from build123d import *

# Parameters (mm, degrees)
SKETCH1_R           = 6.25
SKETCH1_R_2         = 4
BOSS_EXTRUDE1_DEPTH = 15
BOSS_EXTRUDE2_START = 15
SKETCH1_3_R         = 4
BOSS_EXTRUDE2_DEPTH = 30
SKETCH2_R           = 2
CUT_EXTRUDE1_DEPTH  = 12


with BuildPart() as part:
    # Sketch1 → Boss-Extrude1 (new body)
    # profile 1 of 2: a face of its own
    with BuildSketch(Plane.XY):
        Circle(SKETCH1_R)
        Circle(SKETCH1_R_2, mode=Mode.SUBTRACT)
    # profile 2 of 2: a face of its own
    with BuildSketch(Plane.XY):
        Circle(SKETCH1_R_2)
    extrude(amount=BOSS_EXTRUDE1_DEPTH)

    # Sketch1<3> → Boss-Extrude2 (add)
    with BuildSketch(Plane.XY.offset(BOSS_EXTRUDE2_START)):
        Circle(SKETCH1_3_R)
    extrude(amount=BOSS_EXTRUDE2_DEPTH)

    # Sketch2 → Cut-Extrude1 (cut)
    with BuildSketch(Plane(origin=(0, 0, 0), x_dir=(-1, 0, 0), z_dir=(0, 0, -1))):
        Circle(SKETCH2_R)
    extrude(amount=-CUT_EXTRUDE1_DEPTH, mode=Mode.SUBTRACT)


solid = part.part
Part model, mm, in its own coordinate system. A direction names the side the tool comes from. Coordinates: 2 decimals unless noted, no trailing zeros. Loops run counter-clockwise (first coordinate to the right, second up) from the corner with the lowest first, then second, coordinate; pieces in that order, holes last. Notation, with made-up numbers: M 11.25,5 L 67.25,5 A21 ccw 67.25,23 Z; hole C 37,68.25 d3. An arc over 180 degrees is marked long. Use a Markdown table: item, result. Add a question column.
Q1. Cut at C-C (z = 9.5). Write the cut outline in (x, y), and give its area (3 significant figures).
Q2. Probe L1, parallel to Y at x = 0, z = 6.25; L2, parallel to Z at x = -4.25, y = 3.5; L3, parallel to Z at x = 0.75, y = -1.75. List the from-to ranges inside material, lowest first.
Q3. Which spindle directions (+Z, -Z, +X, -X, +Y, -Y) get a long thin tool onto all of the face, cutting with end or side? Do faces 1 (the flat face through (1.3, -4.1, 15)), 2 (the cylindrical face through (0, -2, 6)), 3 (the flat face through (0, -3, 0)). Say none if no direction does.
Q4. Cut at D-D (z = 35.5). Write the cut outline in (x, y), and give its area (3 significant figures).
Q5. Mould opens along X. For faces 4 (the flat face through (0, 0, 12)), 5 (the cylindrical face through (-0.867, -3.905, 29.79)), 6 (the flat face through (0, 0, 45)) say: +X half, -X half, draft (parallel to the pull), parting line (faces both ways), or undercut.
Q6. Cut at A-A (x = 0). Write the cut outline in (y, z), and give its area (4 significant figures).
Q7. Pin check, flat tips, straight feed: P1, Ø3, axis at x = -3, z = 24.5, coming from the -Y side; P2, Ø2, axis at y = -4.5, z = 16.5, coming from the +X side; P3, Ø4, axis at y = 0, z = 35.5, coming from the +X side. Stop position of each tip, or through.
Worked out:
| question | item | result |
|---|---|---|
| 1 | outline | C 0,0 d12.5; hole C 0,0 d4 |
| 1 | area | 110 mm2 |
| 2 | L1 | y = -6.25 to -2, 2 to 6.25 |
| 2 | L2 | z = 0 to 15 |
| 2 | L3 | z = 12 to 45 |
| 3 | face 1 | +Z |
| 3 | face 2 | -Z |
| 3 | face 3 | -Z, +X, -X, +Y, -Y |
| 4 | outline | C 0,0 d8 |
| 4 | area | 50.3 mm2 |
| 5 | face 4 | undercut |
| 5 | face 5 | parting line |
| 5 | face 6 | draft |
| 6 | outline | M -6.25,0 L -2,0 L -2,12 L 2,12 L 2,0 L 6.25,0 L 6.25,15 L 4,15 L 4,45 L -4,45 L -4,15 L -6.25,15 Z |
| 6 | area | 379.5 mm2 |
| 7 | P1 | stops at y = -3.71 |
| 7 | P2 | stops at x = 1.94 |
| 7 | P3 | stops at x = 4 |
